Verification items for the finished model (mm, model axes). Give positions to 0.01 mm unless a question says otherwise; leave off trailing zeros. Write each loop counter-clockwise with the first axis right and the second up, starting at its lowest first coordinate (ties: lowest second). Pieces come first, ordered by that corner, then holes.
Autodesk Inventor part; units mm, degrees
ref_plane "YZ Plane" through (0, 0, 0) normal (1, 0, 0) x (0, 1, 0)
ref_plane "XZ Plane" through (0, 0, 0) normal (0, 1, 0) x (-1, 0, 0)
ref_plane "XY Plane" through (0, 0, 0) normal (0, 0, 1) x (1, 0, 0)
sketch "Sketch1" plane through (0, 0, 0) normal (0, 0, 1) x (1, 0, 0)
  line L0 (-82.55, 12.7) -> (82.55, 12.7)
  line L1 (82.55, 12.7) -> (82.55, -12.7)
  line L2 (82.55, -12.7) -> (-82.55, -12.7)
  line L3 (-82.55, -12.7) -> (-82.55, 12.7)
  line L4 (-82.55, 12.7) -> (82.55, -12.7) construction
  line L5 (82.55, 12.7) -> (-82.55, -12.7) construction
  circle A0 centre (-69.85, 0) radius 5.2705
  circle A1 centre (69.85, 0) radius 5.2705
  point P0 (0, 0)
  dimension "d0" = 165.1
  dimension "d1" = 25.4
  dimension "d2" = 10.541
  dimension "d3" = 12.7
  dimension "d5" = 12.7
extrude "Extrusion1" add sketch "Sketch1" along normal mid plane 12.7
properties part number "connectingRod-4-in"
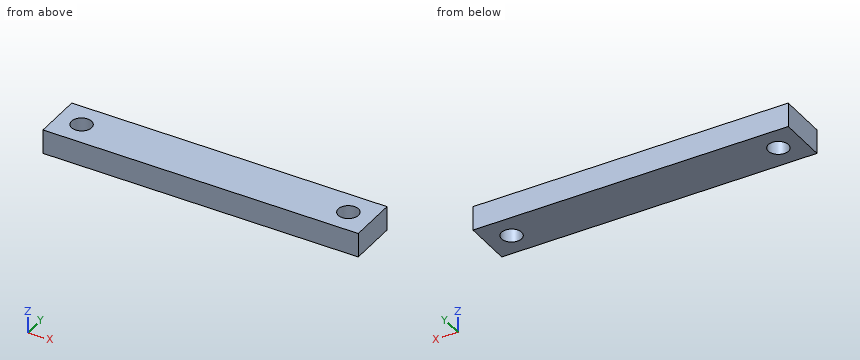
Item 1: Scan lines: line 1 along X through (y, z) = (0.25, 2.75); line 2 along Y through (x, z) = (-69.85, -1); line 3 along X through (y, z) = (-2.5, -2.25). Record each from-to range of solid material in increasing order.
Answer key:
line 1: x = -82.55 to -75.11, -64.59 to 64.59, 75.11 to 82.55
line 2: y = -12.7 to -5.27, 5.27 to 12.7
line 3: x = -82.55 to -74.49, -65.21 to 65.21, 74.49 to 82.55
Item 2: Depth check by flat-ended pin: pin 1 (12 mm diameter, centred on x = -69.85, y = 0, fed in from +Z); pin 2 (9.5 mm diameter, centred on x = 69.85, y = 0, fed in from +Z). Enter the tip coordinate at first touch or a pass-through.
Answer key:
pin 1: stops at z = 6.35
pin 2: passes through
Item 3: Sectioned sample at C-C on z = -1.75. Record the cut outline in (x, y).
Answer key:
outline: (-82.55, -12.7) - (82.55, -12.7) - (82.55, 12.7) - (-82.55, 12.7) - close; hole circle Ø10.54 at (-69.85, 0); hole circle Ø10.54 at (69.85, 0)
Item 4: Sectioned sample at A-A on y = 0. Record the cut outline in (x, z).
Answer key:
outline: (-82.55, -6.35) - (-75.12, -6.35) - (-75.12, 6.35) - (-82.55, 6.35) - close; (-64.58, -6.35) - (64.58, -6.35) - (64.58, 6.35) - (-64.58, 6.35) - close; (75.12, -6.35) - (82.55, -6.35) - (82.55, 6.35) - (75.12, 6.35) - close
Item 5: Sectioned sample at B-B on x = 69.85. Record the cut outline in (y, z), then the cut area to 3 significant figures.
Answer key:
outline: (-12.7, -6.35) - (-5.27, -6.35) - (-5.27, 6.35) - (-12.7, 6.35) - close; (5.27, -6.35) - (12.7, -6.35) - (12.7, 6.35) - (5.27, 6.35) - close
area: 189 mm2
